Design review of the part built by this model. Coordinates are the model's own, in mm. A direction names the side the tool comes from. Round coordinates to 2 decimals unless told otherwise and drop trailing zeros. Write each loop counter-clockwise with the first axis right and the second up, starting at its lowest first coordinate (ties: lowest second). Pieces come first, ordered by that corner, then holes. Notation, with made-up numbers: M -18,59 L 24,59 A7 ccw 24,70 Z; hole C 12,83 d5. An arc over 180 degrees is marked long. One line per question, with ' | ' between items. Start each with the question number.
Item 1: Add section A-A, the plane z = 1.8. State the section outline as (x, y) points, and give its area (3 significant figures).
Item 2: Draft analysis for pull direction Y (two halves, no side actions). For faces 1 (the face through (10.2, 0, 3.5)), 2 (the face through (5.526, 14.102, 1.972)), 3 (the face through (10.2, 16.5, 3.5)), 4 (the face through (14, 4.25, 1)), state which applies: released by +Y, released by -Y, zero draft, split by the parting line, or undercut.
Item 3: Insertion check: pin 1 Ø0.9 at (x, z) = (14.5, 1.5) entering from +Y; pin 2 Ø0.9 at (x, z) = (13.5, 1) entering from -Y; pin 3 Ø2.5 at (x, y) = (7, 12.75) entering from -Z; pin 4 Ø0.9 at (y, z) = (7, 2) entering from +X. Each pin has a flat end and moves straight along its axis. Give the tip position at first contact, or say it passes through.
Item 4: Add section B-B, the plane x = 7. State the section outline as (y, z) points, and give its area (3 significant figures).
Item 5: Add section C-C, the plane y = 12.75. State the section outline as (x, z) points, and give its area (3 significant figures).
Item 6: Machinability: for faces 5 (the face through (14, 1, 1)), 6 (the face through (14, 12.25, 1)), 7 (the face through (12, 14, 1)), 8 (the face through (4.5, 8, 2)), 9 (the face through (7, 15.5, 1)), which of the approach directions +Z, -Z, +X, -X, +Y, -Y give a long, thin tool a straight path to every point of the face, cutting with its end or side? Answer none if there is none.
Item 7: For L1, parallel to Y at x = 7, z = 2.6; L2, parallel to X at y = 12.75, z = 0.8; L3, parallel to Y at x = 14.5, z = 1.25, list the stretches that pass through material, from the lowest coordinate up.
Item 8: Add section D-D, the plane x = 12.5. State the section outline as (y, z) points.
```python
from build123d import *

# Parameters (mm, degrees)
CYLINDER002_R     = 2
CYLINDER002_DEPTH = 20
ARRAY003_Y_COUNT  = 2
ARRAY003_Y_PITCH  = 9
BOX008_W          = 5
BOX008_H          = 8
BOX008_DEPTH      = 3
BOX006_W          = 5
BOX006_H          = 14.5
BOX006_DEPTH      = 3
BOX007_W          = 4
BOX007_H          = 14.5
BOX007_DEPTH      = 3
BOX005_W          = 11.5
BOX005_H          = 16.5
BOX005_DEPTH      = 1


with BuildPart() as hole_array_copy:
    # Cylinder002 → Cylinder002 (new body)
    with BuildSketch(Plane(origin=(7, 3.75, 0), x_dir=(1, 0, 0), z_dir=(0, 0, 1))):
        Circle(CYLINDER002_R)
    extrude(amount=CYLINDER002_DEPTH)

    # Array003 Y: hole array copy ×2


with BuildPart() as hole_array_copy_1:
    add(hole_array_copy.part)
    with Locations(*[(0, i * ARRAY003_Y_PITCH, 0) for i in range(1, ARRAY003_Y_COUNT)]):
        add(hole_array_copy.part)


with BuildPart() as protector_extraction_fusion:
    # Box008 → Box008 (new body)
    with BuildSketch(Plane(origin=(12, 4.25, 0), x_dir=(1, 0, 0), z_dir=(0, 0, 1))):
        with Locations((2.5, 4)):
            Rectangle(BOX008_W, BOX008_H)
    extrude(amount=BOX008_DEPTH)

    # Fusion002: union hole array copy
    add(hole_array_copy_1.part)


with BuildPart() as hole_stand_cube001:
    # Box006 → Box006 (new body)
    with BuildSketch(Plane(origin=(4.5, 1, 0), x_dir=(1, 0, 0), z_dir=(0, 0, 1))):
        with Locations((2.5, 7.25)):
            Rectangle(BOX006_W, BOX006_H)
    extrude(amount=BOX006_DEPTH)


with BuildPart() as usb_side_protection_cube:
    # Box007 → Box007 (new body)
    with BuildSketch(Plane(origin=(12, 1, 0), x_dir=(1, 0, 0), z_dir=(0, 0, 1))):
        with Locations((2, 7.25)):
            Rectangle(BOX007_W, BOX007_H)
    extrude(amount=BOX007_DEPTH)


with BuildPart() as protector_cut:
    # Box005 → Box005 (new body)
    with BuildSketch(Plane(origin=(4.5, 0, 3), x_dir=(1, 0, 0), z_dir=(0, 0, 1))):
        with Locations((5.75, 8.25)):
            Rectangle(BOX005_W, BOX005_H)
    extrude(amount=BOX005_DEPTH)

    # Fusion001: union hole stand cube001, usb side protection cube
    add(hole_stand_cube001.part)
    add(usb_side_protection_cube.part)

    # Cut003: cut protector extraction fusion
    add(protector_extraction_fusion.part, mode=Mode.SUBTRACT)


solid = protector_cut.part
```
Computed values:
1) outline: M 4.5,1 L 9.5,1 L 9.5,15.5 L 4.5,15.5 Z; M 12,1 L 16,1 L 16,4.25 L 12,4.25 Z; M 12,12.25 L 16,12.25 L 16,15.5 L 12,15.5 Z; hole C 7,3.75 d4; hole C 7,12.75 d4 | area: 73.4 mm^2
2) face 1: released by -Y | face 2: undercut | face 3: released by +Y | face 4: undercut
3) pin 1: stops at y = 15.5 | pin 2: stops at y = 1 | pin 3: passes through | pin 4: stops at x = 9.5
4) outline: M 0,3 L 1,3 L 1,0 L 1.75,0 L 1.75,4 L 0,4 Z; M 5.75,0 L 10.75,0 L 10.75,4 L 5.75,4 Z; M 14.75,0 L 15.5,0 L 15.5,3 L 16.5,3 L 16.5,4 L 14.75,4 Z | area: 28.0 mm^2
5) outline: M 4.5,0 L 5,0 L 5,4 L 4.5,4 Z; M 9,0 L 9.5,0 L 9.5,3 L 12,3 L 12,0 L 16,0 L 16,4 L 9,4 Z | area: 22.5 mm^2
6) face 5: -Z, +X, -X, -Y | face 6: -Z, +X | face 7: -Z, +Y, -Y | face 8: +Z, -Z, -X, +Y, -Y | face 9: -Z, +X, -X, +Y
7) L1: y = 1 to 1.75, 5.75 to 10.75, 14.75 to 15.5 | L2: x = 4.5 to 5, 9 to 9.5, 12 to 16 | L3: y = 1 to 4.25, 12.25 to 15.5
8) outline: M 0,3 L 1,3 L 1,0 L 4.25,0 L 4.25,3 L 12.25,3 L 12.25,0 L 15.5,0 L 15.5,3 L 16.5,3 L 16.5,4 L 0,4 Z
